Model file for the job. Use its own axes, mm. Give positions to 0.01 mm unless a question says otherwise; leave off trailing zeros. Loops run counter-clockwise (first coordinate to the right, second up) from the corner with the lowest first, then second, coordinate; pieces in that order, holes last. Notation, with made-up numbers: M 38,-16 L 76,-16 A32 cw 76,16 Z; hole C 17.25,19.25 d11. An arc over 180 degrees is marked long. Use CSV: the item, a comma, the result in double quotes. Start each with the question number.
(1) Slice it at A-A on z = 27.5. List the corners of the cut face in (x, y), and give its area (3 significant figures).
(2) Wall check: line 1 along Y through (x, z) = (21, 48.5); line 2 along X through (y, z) = (-48.4, 27); line 3 along X through (y, z) = (-47.5, 9.5). Give the ranges that are in metal, low to high. Write a range as from..to.
(3) Two-plate mould, pull along X, no slides. Class faces 1 (the face through (21.1, -45.8, 55)), 2 (the face through (-9.5, -48, 27)), 3 (the face through (21, -49, 6)), 4 (the face through (52.5, -48, 27)): pulls with the +X half, pulls with the -X half, needs draft (parallel to the pull), parting line crosses it, or undercut.
(4) Slice it at B-B on x = 21. List the corners of the cut face in (y, z), and give its area (3 significant figures).
(5) Slice it at C-C on y = -47.5. List the corners of the cut face in (x, z), and give its area (3 significant figures).
(6) Slice it at D-D on z = 51.5. List the corners of the cut face in (x, y).
```python
from build123d import *

# Parameters (mm, degrees)
ESQUISSE1_W             = 62
ESQUISSE1_H             = 5
BOSS_EXTRU_1_DEPTH      = 55
ESQUISSE2_R             = 15
ENL_V_MAT_EXTRU_1_DEPTH = 6
ESQUISSE5_R             = 1.5
ENL_V_MAT_EXTRU_4_DEPTH = 56


with BuildPart() as part:
    # Esquisse1 → Boss.-Extru.1 (new body)
    with BuildSketch(Plane.XY):
        with Locations((21.5, -47.5)):
            Rectangle(ESQUISSE1_W, ESQUISSE1_H)
    extrude(amount=BOSS_EXTRU_1_DEPTH)

    # Esquisse2 → Enlèv. mat.-Extru.1 (cut, through all)
    with BuildSketch(Plane(origin=(0, -45, 0), x_dir=(-1, 0, 0), z_dir=(0, 1, 0))):
        with Locations((-21.5, 27.5)):
            Circle(ESQUISSE2_R)
    extrude(amount=-ENL_V_MAT_EXTRU_1_DEPTH, mode=Mode.SUBTRACT)

    # Esquisse5 → Enlèv. mat.-Extru.4 (cut, through all)
    with BuildSketch(Plane.XY.offset(55)):
        with Locations((21, -47.5)):
            Circle(ESQUISSE5_R)
    extrude(amount=-ENL_V_MAT_EXTRU_4_DEPTH, mode=Mode.SUBTRACT)


solid = part.part
```
Reply:
1,outline,"M -9.5,-50 L 6.5,-50 L 6.5,-45 L -9.5,-45 Z; M 36.5,-50 L 52.5,-50 L 52.5,-45 L 36.5,-45 Z"
1,area,"160 mm^2"
2,line 1,"y = -50..-49, -46..-45"
2,line 2,"x = -9.5..6.51, 36.49..52.5"
2,line 3,"x = -9.5..19.5, 22.5..52.5"
3,face 1,"needs draft"
3,face 2,"pulls with the -X half"
3,face 3,"undercut"
3,face 4,"pulls with the +X half"
4,outline,"M -50,0 L -49,0 L -49,12.51 L -50,12.51 Z; M -50,42.49 L -49,42.49 L -49,55 L -50,55 Z; M -46,0 L -45,0 L -45,12.51 L -46,12.51 Z; M -46,42.49 L -45,42.49 L -45,55 L -46,55 Z"
4,area,"50.0 mm^2"
5,outline,"M -9.5,0 L 19.5,0 L 19.5,12.63 A15 cw 19.5,42.37 L 19.5,55 L -9.5,55 Z; M 22.5,0 L 52.5,0 L 52.5,55 L 22.5,55 L 22.5,42.47 A15 cw 22.5,12.53 Z"
5,area,"2,630 mm^2"
6,outline,"M -9.5,-50 L 52.5,-50 L 52.5,-45 L -9.5,-45 Z; hole C 21,-47.5 d3"
